Geometry: final body of the model. Coordinates: model frame, mm. Give positions to 0.01 mm unless a question says otherwise; leave off trailing zeros. Loops run counter-clockwise (first coordinate to the right, second up) from the corner with the lowest first, then second, coordinate; pieces in that order, holes last. Notation, with made-up numbers: (13, 45.5) -> (53, 45.5) arc R15 ccw to (53, 58.5) -> close; hole circle Ø11 at (-38, 55). An arc over 180 degrees is marked (long way). Answer in a Markdown table with one row per item. Add a question column.
1) Section query C-C (x = 104). Return the cut outline in (y, z), plus the area to 3 significant figures.
2) Line query: line 1 (X direction, y = 1.7, z = 14); line 2 (Z direction, x = -129.5, y = 0.65); line 3 (Z direction, x = 107, y = 2.15). Output: solid intervals per line, ascending. Write a range as from..to.
3) First-contact query: P1, Ø0.8, axis at y = 1, z = 13.5, coming from the -X side; P2, Ø1, axis at y = 2, z = 15.5, coming from the +X side. Flat tips, straight axial feed; report the tip coordinate or a pass-through.
4) Section query B-B (y = 1.5). Return the cut outline in (x, z), plus the area to 3 significant figures.
5) Section query A-A (x = -8.5). Return the cut outline in (y, z), plus the area to 3 significant figures.
```python
from build123d import *

# Parameters (mm, degrees)
SKETCH1_W           = 60
SKETCH1_H           = 3.218
BOSS_EXTRUDE1_DEPTH = 2.7


with BuildPart() as part:
    # Sketch1 → Boss-Extrude1 (new body)
    with BuildSketch(Plane(origin=(0, 0, 0), x_dir=(1, 0, 0), z_dir=(0, 1, 0))):
        Polygon((-150, -14.79), (-90, -14.79), (-90, -11.572), (-150, -11.572), (-150, 30), (150, 30), (150, -14.79), (90, -14.79), (90, -16.782), (150, -16.782), (150, -30), (-150, -30), align=None)
        with Locations((0, -13.181)):
            Rectangle(SKETCH1_W, SKETCH1_H, mode=Mode.SUBTRACT)
    extrude(amount=BOSS_EXTRUDE1_DEPTH)


solid = part.part
```
Evaluation:
| question | item | result |
|---|---|---|
| 1 | outline | (0, -30) -> (2.7, -30) -> (2.7, 14.79) -> (0, 14.79) -> close; (0, 16.78) -> (2.7, 16.78) -> (2.7, 30) -> (0, 30) -> close |
| 1 | area | 157 mm² |
| 2 | line 1 | -90..-30, 30..150 |
| 2 | line 2 | -30..11.57, 14.79..30 |
| 2 | line 3 | -30..14.79, 16.78..30 |
| 3 | P1 | x = -90 |
| 3 | P2 | x = 90 |
| 4 | outline | (-150, -30) -> (150, -30) -> (150, 14.79) -> (90, 14.79) -> (90, 16.78) -> (150, 16.78) -> (150, 30) -> (-150, 30) -> (-150, 14.79) -> (-90, 14.79) -> (-90, 11.57) -> (-150, 11.57) -> close; hole (-30, 11.57) -> (30, 11.57) -> (30, 14.79) -> (-30, 14.79) -> close |
| 4 | area | 17,500 mm² |
| 5 | outline | (0, -30) -> (2.7, -30) -> (2.7, 11.57) -> (0, 11.57) -> close; (0, 14.79) -> (2.7, 14.79) -> (2.7, 30) -> (0, 30) -> close |
| 5 | area | 153 mm² |
